```python
from build123d import *

# Parameters (mm, degrees)
SKETCH1_R                = 45
SKETCH1_R_2              = 1.6
BOSS_EXTRUDE1_DEPTH      = 5
SKETCH4_R                = 36.501480924
CUT_EXTRUDE1_DEPTH       = 3
SKETCH5_R                = 36.501480924
CUT_EXTRUDE2_DEPTH       = 3
SKETCH2_R                = 3
SKETCH2_R_2              = 1.6
BOSS_EXTRUDE2_DEPTH      = 4.8
BOSS_EXTRUDE2_DEPTH_BACK = 4
CUT_EXTRUDE3_DEPTH       = 10
CIRPATTERN1_COUNT        = 9


with BuildPart() as part:
    # Sketch1 → Boss-Extrude1 (new body, symmetric)
    with BuildSketch(Plane(origin=(0, 0, 0), x_dir=(1, 0, 0), z_dir=(0, 1, 0))):
        with Locations((0, -0.088724957)):
            Circle(SKETCH1_R)
        with Locations((0, -0.088724957)):
            Circle(SKETCH1_R_2, mode=Mode.SUBTRACT)
    extrude(amount=BOSS_EXTRUDE1_DEPTH, both=True)

    # Sketch4 → Cut-Extrude1 (cut)
    with BuildSketch(Plane(origin=(0, 5, 0), x_dir=(1, 0, 0), z_dir=(0, 1, 0))):
        Circle(SKETCH4_R)
    extrude(amount=-CUT_EXTRUDE1_DEPTH, mode=Mode.SUBTRACT)

    # Sketch5 → Cut-Extrude2 (cut)
    with BuildSketch(Plane.XZ.offset(5)):
        Circle(SKETCH5_R)
    extrude(amount=-CUT_EXTRUDE2_DEPTH, mode=Mode.SUBTRACT)

    # Sketch2 → Boss-Extrude2 (add, two sides)
    with BuildSketch(Plane.XZ.offset(5)) as boss_extrude2_sk:
        Circle(SKETCH2_R)
        with Locations((0, 0.088724957)):
            Circle(SKETCH2_R_2, mode=Mode.SUBTRACT)
    extrude(amount=BOSS_EXTRUDE2_DEPTH)
    extrude(boss_extrude2_sk.sketch, amount=-BOSS_EXTRUDE2_DEPTH_BACK)

    # Sketch6 → Cut-Extrude3 (cut)
    with BuildSketch(Plane.XZ.offset(2)):
        with BuildLine():
            ThreePointArc((7.771439261, 35.664588059), (-0.52889107, 36.497649018), (-8.801597259, 35.424426535))
            add(Edge.make_bspline(
                [(-8.801597259, 35.424426535), (0.488382971, -15.925400328), (7.771439261, 35.664588059)],
                knots=[0, 0, 0, 1, 1, 1], degree=2))
        make_face()
    cut_extrude3 = extrude(amount=-CUT_EXTRUDE3_DEPTH, mode=Mode.SUBTRACT)

    # CirPattern1: Cut-Extrude3 ×9 about axis
    cirpattern1_axis = Axis((0, 5, 0.088724957), (0, -1, 0))
    for i in range(1, CIRPATTERN1_COUNT):
        add(cut_extrude3.rotate(cirpattern1_axis, i * 360 / CIRPATTERN1_COUNT), mode=Mode.SUBTRACT)


solid = part.part
```
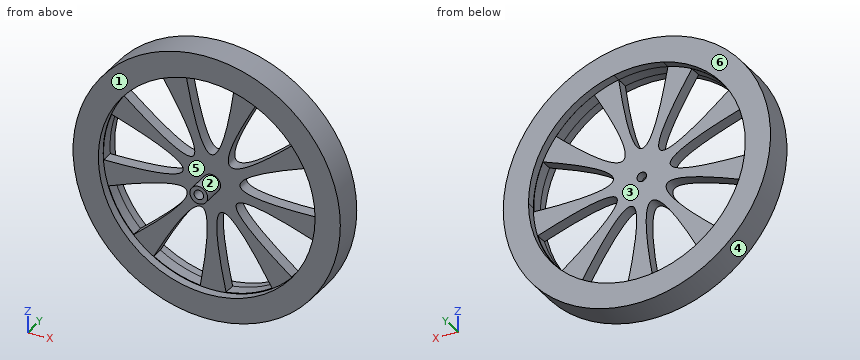
Verification items for the finished model (mm, model axes). Face numbers are marked on the shaded views. A direction names the side the tool comes from. Give positions to 0.01 mm unless a question says otherwise; leave off trailing zeros. Write each loop counter-clockwise with the first axis right and the second up, starting at its lowest first coordinate (ties: lowest second). Pieces come first, ordered by that corner, then holes. Notation, with made-up numbers: M -26.75,-18.5 L 4.25,-18.5 A7 cw 4.25,-11.5 Z; hole C 70,13.25 d9. An arc over 180 degrees is marked long. One line per question, with ' | ' between items.
1) Thickness scan on line 1 along Z through (x, y) = (0, -3.35); line 2 along Z through (x, y) = (0, -1.35); line 3 along Z through (x, y) = (0, -8.35). Record the ranges inside material, lowest first. Write a range as [from, to].
Result:
line 1: z = [-44.91, -36.5], [-3, -1.51], [1.69, 3], [36.5, 45.09] | line 2: z = [-44.91, -1.51], [1.69, 9.81], [36.5, 45.09] | line 3: z = [-3, -1.51], [1.69, 3]
2) Section check A-A on z = -33. State how many separate pieces and enclosed holes the cut face has, plus the area to 3 significant figures.
Result:
separate pieces: 3 | enclosed holes: 0 | area: 331 mm2
3) Set-up check for the marked faces 5 and 6: record each of +Z, -Z, +X, -X, +Y, -Y from which the full face is reachable in a straight line by a thin tool's end or side.
Result:
face 5: -Y | face 6: +Z, -Z, +X, -X, +Y
4) Section check B-B on y = -7. Enter the section's corners in (x, z).
Result:
outline: C 0,0 d6; hole C 0,0.09 d3.2
5) Mould release check, pull along X, two halves, no side actions. Record for the marked faces 1, 2, 3 and 4: released by +X, released by -X, zero draft, split by the parting line, or undercut.
Result:
face 1: zero draft | face 2: undercut | face 3: undercut | face 4: split by the parting line
6) Gauge pin test, flat ends, axial feed: pin 1 Ø1.5 at (x, y) = (-4.5, -7) entering from +Z; pin 2 Ø3 at (x, y) = (11, -0.5) entering from +Z; pin 3 Ø5 at (y, z) = (-1, 23.5) entering from -X; pin 4 Ø5 at (x, z) = (-35.5, -12) entering from -Y. Record the tip position at first contact, or that the pin passes through.
Result:
pin 1: passes through | pin 2: stops at z = 44.07 | pin 3: stops at x = -39.85 | pin 4: stops at y = -5
